Source: CAD feature listing. Evaluate the final solid. Frame: model axes, mm. Face numbers are marked on the shaded views. Give positions to 0.01 mm unless a question says otherwise; leave off trailing zeros. Write item = value, one per line.
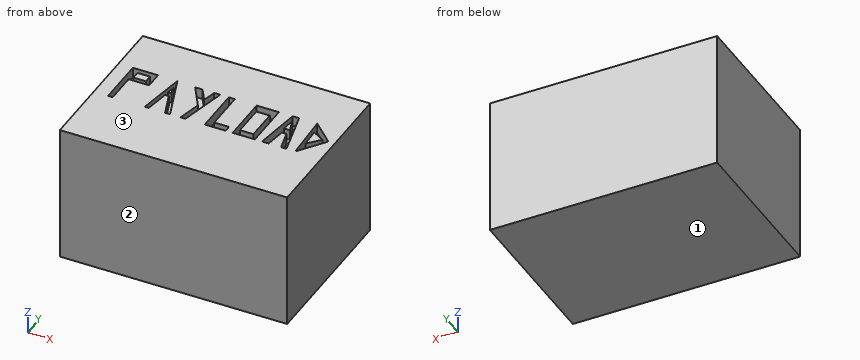
from build123d import *

# Parameters (mm, degrees)
SKETCH1_W           = 558.8
SKETCH1_H           = 398.78
BOSS_EXTRUDE1_DEPTH = 339.852
SKETCH2_W           = 30.678718516
SKETCH2_H           = 19.85093551
SKETCH2_W_2         = 54.740458529
SKETCH2_H_2         = 115.513846454
SKETCH2_W_3         = 33.084892517
SKETCH2_H_3         = 78.80219854
CUT_EXTRUDE1_DEPTH  = 25.4


with BuildPart() as part:
    # Sketch1 → Boss-Extrude1 (new body)
    with BuildSketch(Plane.XY):
        Rectangle(SKETCH1_W, SKETCH1_H)
    extrude(amount=-BOSS_EXTRUDE1_DEPTH)

    # Sketch2 → Cut-Extrude1 (cut)
    # profile 1 of 7: a face of its own
    with BuildSketch(Plane.XY):
        Polygon((-244.226661127, 82.712231293), (-244.226661127, -36.393381769), (-232.797334621, -36.393381769), (-232.797334621, 40.002642771), (-182.267680595, 40.002642771), (-182.267680595, 82.712231293), align=None)
        with Locations((-210.840996859, 60.154350031)):
            Rectangle(SKETCH2_W, SKETCH2_H, mode=Mode.SUBTRACT)
    # profile 2 of 7: a face of its own
    with BuildSketch(Plane.XY):
        Polygon((-153.99513608, -36.393381769), (-134.74574407, 82.712231293), (-92.036155548, -36.393381769), (-104.067025554, -36.393381769), (-125.421819815, 23.159424762), (-134.74574407, 23.159424762), (-144.370440075, -36.393381769), align=None)
        Polygon((-130.083781942, 56.244317279), (-133.454387424, 35.388695861), (-125.421819815, 35.388695861), align=None, mode=Mode.SUBTRACT)
    # profile 3 of 7: a face of its own
    with BuildSketch(Plane.XY):
        Polygon((-27.74569837, 79.120464685), (-54.138915028, -36.393381769), (-66.169785034, -36.393381769), (-52.973176705, 21.363541458), (-89.245743132, 79.120464685), (-71.109459919, 79.120464685), (-50.193871527, 45.81650657), (-42.584406436, 79.120464685), align=None)
    # profile 4 of 7: a face of its own
    with BuildSketch(Plane.XY):
        Polygon((-6.616978503, 79.120464685), (-6.616978503, -36.393381769), (44.683403133, -36.393381769), (44.683403133, -20.15170726), (8.421609004, -20.15170726), (8.421609004, 79.120464685), align=None)
    # profile 5 of 7: a face of its own
    with BuildSketch(Plane.XY):
        with Locations((89.329209797, 21.363541458)):
            Rectangle(SKETCH2_W_2, SKETCH2_H_2)
        with Locations((88.126122796, 19.24939201)):
            Rectangle(SKETCH2_W_3, SKETCH2_H_3, mode=Mode.SUBTRACT)
    # profile 6 of 7: a face of its own
    with BuildSketch(Plane.XY):
        Polygon((150.385875078, 79.120464685), (134.14420057, -36.393381769), (150.385875078, -36.393381769), (157.386476137, 13.396210762), (169.033723588, 13.396210762), (181.064593594, -36.393381769), (194.298550601, -36.393381769), (166.386450903, 79.120464685), align=None)
        Polygon((158.386162991, 61.658208782), (153.886175607, 29.653451429), (169.033723588, 29.653451429), align=None, mode=Mode.SUBTRACT)
    # profile 7 of 7: a face of its own
    with BuildSketch(Plane.XY):
        Polygon((210.874736117, 79.120464685), (215.954116612, -36.393381769), (263.476053137, 29.653451429), align=None)
        Polygon((220.207882974, 46.326740486), (222.244964668, 0), (249.039009129, 29.653451429), align=None, mode=Mode.SUBTRACT)
    extrude(amount=-CUT_EXTRUDE1_DEPTH, mode=Mode.SUBTRACT)


solid = part.part
1) Contact query for a flat-ended pin moving along its axis: pin 1 (3 mm diameter, centred on x = 32, y = -27.5, fed in from +Z). Output: stop coordinate, or through.
Computed:
pin_1 = -25.4
2) Draft query along Z for the marked faces 1, 2 and 3. Return one class per face: pulls with the +Z half, pulls with the -Z half, needs draft (parallel to the pull), parting line crosses it, or undercut.
Computed:
face_1 = pulls with the -Z half
face_2 = needs draft
face_3 = pulls with the +Z half
3) Material intervals for L1, parallel to Z at x = -242, y = 77.5, sorted ascending.
Computed:
L1 = -339.85 to -25.4
